Verification items for the finished model (mm, model axes). A direction names the side the tool comes from. Coordinates: 2 decimals unless noted, no trailing zeros. Loops run counter-clockwise (first coordinate to the right, second up) from the corner with the lowest first, then second, coordinate; pieces in that order, holes last. Notation, with made-up numbers: (26.5, 20) -> (33.5, 20) arc R22 ccw to (33.5, 44) -> close; hole circle Ø10 at (-39, -38). An arc over 180 degrees is marked (long way). Answer as a JSON object with one key per item and string values. Group by question number.
Q1. Cross-section at B-B on z = 0.9. Record the boundary of the cut face in (x, y), and give its area (3 significant figures).
Q2. Set-up check for faces 1 (the flat face through (11, -11, 6)), 2 (the cylindrical face through (19.226, 8.351, 5.014)): record each of +Z, -Z, +X, -X, +Y, -Y from which the full face is reachable in a straight line by a thin tool's end or side.
Q3. Cross-section at D-D on y = -9.5. Give the number of separate pieces and of enclosed holes in the cut face, and give its area (3 significant figures).
Q4. Gauge pin test, flat ends, axial feed: pin 1 Ø7 at (x, y) = (0, 19) entering from +Z; pin 2 Ø1 at (y, z) = (-5.5, 1.5) entering from -X; pin 3 Ø3.5 at (x, y) = (0, -19) entering from +Z; pin 4 Ø3 at (x, z) = (7.5, 0.5) entering from -Y. Record the tip position at first contact, or that the pin passes through.
Q5. Scan lines: L1, parallel to Y at x = 0, z = 2.65; L2, parallel to Y at x = -19, z = 5.3; L3, parallel to Y at x = -15, z = 1.4. Record each from-to range of solid material in increasing order.
Q6. Release check for a two-part mould opening along Y. For faces 3 (the cylindrical face through (17.98, 8.87, 1.97)), 4 (the flat face through (12, -6, 0)) record: released by +Y, released by -Y, zero draft, split by the parting line, or undercut.
Q7. Cross-section at C-C on x = 0. Record the boundary of the cut face in (y, z).
Q8. Cross-section at A-A on y = 0. Record the boundary of the cut face in (x, z).
```python
from build123d import *

# Parameters (mm, degrees)
SKETCH1_R           = 27
SKETCH1_R_2         = 1.65
SKETCH1_R_3         = 12.5
BOSS_EXTRUDE1_DEPTH = 6
SKETCH2_R           = 3
CUT_EXTRUDE1_DEPTH  = 2
CHAMFER1_SIZE       = 1


with BuildPart() as part:
    # Sketch1 → Boss-Extrude1 (new body)
    with BuildSketch(Plane.XY):
        Circle(SKETCH1_R)
        with Locations((0, 19)):
            Circle(SKETCH1_R_2, mode=Mode.SUBTRACT)
        with Locations((16.454482672, 9.5)):
            Circle(SKETCH1_R_2, mode=Mode.SUBTRACT)
        with Locations((16.454482672, -9.5)):
            Circle(SKETCH1_R_2, mode=Mode.SUBTRACT)
        with Locations((0, -19)):
            Circle(SKETCH1_R_2, mode=Mode.SUBTRACT)
        with Locations((-16.454482672, -9.5)):
            Circle(SKETCH1_R_2, mode=Mode.SUBTRACT)
        with Locations((-16.454482672, 9.5)):
            Circle(SKETCH1_R_2, mode=Mode.SUBTRACT)
        Circle(SKETCH1_R_3, mode=Mode.SUBTRACT)
    extrude(amount=BOSS_EXTRUDE1_DEPTH)

    # Sketch2 → Cut-Extrude1 (cut)
    with BuildSketch(Plane.XY.offset(6)):
        with Locations((0, 19)):
            Circle(SKETCH2_R)
        with Locations((16.454482672, 9.5)):
            Circle(SKETCH2_R)
        with Locations((16.454482672, -9.5)):
            Circle(SKETCH2_R)
        with Locations((0, -19)):
            Circle(SKETCH2_R)
        with Locations((-16.454482672, -9.5)):
            Circle(SKETCH2_R)
        with Locations((-16.454482672, 9.5)):
            Circle(SKETCH2_R)
    extrude(amount=-CUT_EXTRUDE1_DEPTH, mode=Mode.SUBTRACT)

    # Chamfer1
    chamfer1_edges = [part.edges().sort_by_distance(p)[0] for p in [
        (-27, 0, 6),
        (-12.5, 0, 6),
    ]]
    chamfer(chamfer1_edges, length=CHAMFER1_SIZE)


solid = part.part
```
Computed values:
{
 "1": {"outline": "circle Ø54 at (0, 0); hole circle Ø3.3 at (-16.45, -9.5); hole circle Ø3.3 at (-16.45, 9.5); hole circle Ø25 at (0, 0); hole circle Ø3.3 at (0, -19); hole circle Ø3.3 at (0, 19); hole circle Ø3.3 at (16.45, -9.5); hole circle Ø3.3 at (16.45, 9.5)", "area": "1,750 mm²"},
 "2": {"face 1": "+Z, +X, -X, +Y, -Y", "face 2": "+Z"},
 "3": {"separate pieces": "4", "enclosed holes": "0", "area": "153 mm²"},
 "4": {"pin 1": "stops at z = 6", "pin 2": "stops at x = -26.53", "pin 3": "stops at z = 4", "pin 4": "stops at y = -26.32"},
 "5": {"L1": "y = -27 to -20.65, -17.35 to -12.5, 12.5 to 17.35, 20.65 to 27", "L2": "y = -18.76 to -11.09, -7.91 to 7.91, 11.09 to 18.76", "L3": "y = -22.45 to -10.28, -8.72 to 8.72, 10.28 to 22.45"},
 "6": {"face 3": "undercut", "face 4": "zero draft"},
 "7": {"outline": "(-27, 0) -> (-20.65, 0) -> (-20.65, 4) -> (-22, 4) -> (-22, 6) -> (-26, 6) -> (-27, 5) -> close; (-17.35, 0) -> (-12.5, 0) -> (-12.5, 5) -> (-13.5, 6) -> (-16, 6) -> (-16, 4) -> (-17.35, 4) -> close; (12.5, 0) -> (17.35, 0) -> (17.35, 4) -> (16, 4) -> (16, 6) -> (13.5, 6) -> (12.5, 5) -> close; (20.65, 0) -> (27, 0) -> (27, 5) -> (26, 6) -> (22, 6) -> (22, 4) -> (20.65, 4) -> close"},
 "8": {"outline": "(-27, 0) -> (-12.5, 0) -> (-12.5, 5) -> (-13.5, 6) -> (-26, 6) -> (-27, 5) -> close; (12.5, 0) -> (27, 0) -> (27, 5) -> (26, 6) -> (13.5, 6) -> (12.5, 5) -> close"}
}
